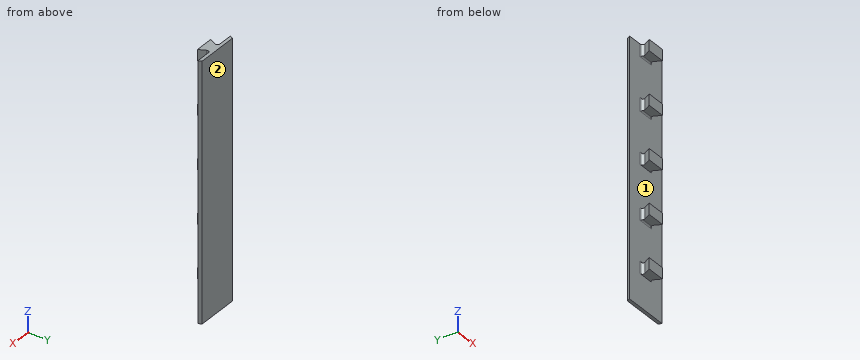
from build123d import *

# Parameters (mm, degrees)
BOSS_EXTRUDE1_DEPTH     = 34.5
CUT_EXTRUDE1_DEPTH      = 59.851529292
CUT_EXTRUDE1_DEPTH_BACK = 59.851529292
SKETCH2_W               = 6.5
SKETCH2_H               = 1.55
BOSS_EXTRUDE2_DEPTH     = 5
FILLET1_R               = 0.2


with BuildPart() as part:
    # Sketch1 → Boss-Extrude1 (new body)
    with BuildSketch(Plane(origin=(0, 0, 0), x_dir=(1, 0, 0), z_dir=(0, 0, -1))):
        with BuildLine():
            Line((-3.5, 46), (-1.217705098, 46))
            ThreePointArc((-1.217705098, 46), (-0.919977315, 46.165994111), (-0.904655581, 46.506524758))
            Line((-0.904655581, 46.506524758), (-1.426393202, 47.55))
            Line((-1.426393202, 47.55), (1.426393202, 47.55))
            Line((1.426393202, 47.55), (0.904655581, 46.506524758))
            ThreePointArc((0.904655581, 46.506524758), (0.919977315, 46.165994111), (1.217705098, 46))
            Line((1.217705098, 46), (3.5, 46))
            Line((3.5, 46), (3.25, 45.5))
            Line((3.25, 45.5), (-3.25, 45.5))
            Line((-3.25, 45.5), (-3.5, 46))
        make_face()
    extrude(amount=BOSS_EXTRUDE1_DEPTH)

    # Sketch2 → Cut-Extrude1 (cut, two sides: drawn at the far end of the back side and taken through both)
    with BuildSketch(Plane(origin=(0, 0, 0), x_dir=(0, 0, -1), z_dir=(1, 0, 0)).offset(-CUT_EXTRUDE1_DEPTH_BACK)):
        with Locations((4.95, -46.775)):
            Rectangle(SKETCH2_W, SKETCH2_H)
        with Locations((29.55, -46.775)):
            Rectangle(SKETCH2_W, SKETCH2_H)
        with Locations((21.35, -46.775)):
            Rectangle(SKETCH2_W, SKETCH2_H)
        with Locations((13.15, -46.775)):
            Rectangle(SKETCH2_W, SKETCH2_H)
    extrude(amount=CUT_EXTRUDE1_DEPTH + CUT_EXTRUDE1_DEPTH_BACK, mode=Mode.SUBTRACT)

    # Sketch3 → Boss-Extrude2 (add)
    with BuildSketch(Plane(origin=(0, 0, -34.5), x_dir=(-1, 0, 0), z_dir=(0, 0, -1))):
        Polygon((1.217705098, -46), (-1.217705098, -46), (-3.5, -46), (-3.25, -45.5), (3.25, -45.5), (3.5, -46), align=None)
    extrude(amount=BOSS_EXTRUDE2_DEPTH)

    # Fillet1
    fillet1_edges = [part.edges().sort_by_distance(p)[0] for p in [
        (0, -46, -26.3),
        (0, -46, -32.8),
        (0, -46, -1.7),
        (0, -46, -8.2),
        (0, -46, -9.9),
        (0, -46, -16.4),
    ]]
    fillet(fillet1_edges, radius=FILLET1_R)


solid = part.part
Verification items for the finished model (mm, model axes). Face numbers are marked on the shaded views. Give positions to 0.01 mm unless a question says otherwise; leave off trailing zeros. Write each loop counter-clockwise with the first axis right and the second up, starting at its lowest first coordinate (ties: lowest second). Pieces come first, ordered by that corner, then holes. Notation, with made-up numbers: M 74,10.25 L 118,10.25 A14 cw 118,25.25 Z; hole C 73.25,49.25 d11. An arc over 180 degrees is marked long. Put each result on its own line as item: value. Start each with the question number.
1. Section check D-D (x = 2). Record the cut outline in (y, z), and give its area (4 significant figures).
2. Draft check along Z on the marked faces 1 and 2. Enter one of: +Z half, -Z half, draft (parallel to the pull), parting line (faces both ways), or undercut.
3. Section check A-A (x = 0.25). Record the cut outline in (y, z).
4. Go/stop test with flat-tipped pins: pin 1 Ø0.5 at (x, y) = (0.5, -47) entering from -Z; pin 2 Ø1 at (x, y) = (-2.5, -47) entering from +Z. Record where each tip stops, or that it passes through.
5. Scan lines: line 1 along Z through (x, y) = (0.25, -46.3); line 2 along Y through (x, z) = (-1.5, -18); line 3 along Y through (x, z) = (1, -9.5). Record each from-to range of solid material in increasing order. Write a range as [from, to].
6. Section check B-B (y = -47.15). Record the cut outline in (x, z).
7. Section check C-C (z = -11.5). Record the cut outline in (x, y), and give its area (4 significant figures).
Answer list:
1. outline: M -46,-39.5 L -45.5,-39.5 L -45.5,0 L -46,0 Z
1. area: 19.75 mm2
2. face 1: undercut
2. face 2: draft
3. outline: M -47.55,-34.5 L -46,-34.5 L -46,-39.5 L -45.5,-39.5 L -45.5,0 L -47.55,0 L -47.55,-1.7 L -46.2,-1.7 A0.2 cw -46,-1.9 L -46,-8 A0.2 cw -46.2,-8.2 L -47.55,-8.2 L -47.55,-9.9 L -46.2,-9.9 A0.2 cw -46,-10.1 L -46,-16.2 A0.2 cw -46.2,-16.4 L -47.55,-16.4 L -47.55,-18.1 L -46,-18.1 L -46,-24.6 L -47.55,-24.6 L -47.55,-26.3 L -46.2,-26.3 A0.2 cw -46,-26.5 L -46,-32.6 A0.2 cw -46.2,-32.8 L -47.55,-32.8 Z
4. pin 1: z = -34.5
4. pin 2: through
5. line 1: [-34.5, -32.8], [-26.3, -24.6], [-18.1, -16.4], [-9.9, -8.2], [-1.7, 0]
5. line 2: [-46, -45.5]
5. line 3: [-47.55, -46.7], [-46.08, -45.5]
6. outline: M -1.23,-34.5 L 1.23,-34.5 L 1.23,-32.8 L -1.23,-32.8 Z; M -1.23,-26.3 L 1.23,-26.3 L 1.23,-24.6 L -1.23,-24.6 Z; M -1.23,-18.1 L 1.23,-18.1 L 1.23,-16.4 L -1.23,-16.4 Z; M -1.23,-9.9 L 1.23,-9.9 L 1.23,-8.2 L -1.23,-8.2 Z; M -1.23,-1.7 L 1.23,-1.7 L 1.23,0 L -1.23,0 Z
7. outline: M -3.5,-46 L 3.5,-46 L 3.25,-45.5 L -3.25,-45.5 Z
7. area: 3.375 mm2
